Build history of the part. All positions in model axes, mm. A direction names the side the tool comes from. Give positions to 0.01 mm unless a question says otherwise; leave off trailing zeros. Loops run counter-clockwise (first coordinate to the right, second up) from the corner with the lowest first, then second, coordinate; pieces in that order, holes last.
1) Wall check: line 1 (Z direction, x = -69.85, y = -1.05); line 2 (Z direction, x = -69, y = -2); line 3 (Z direction, x = 20, y = -34.5). Give the ranges that are in metal, low to high.
2) Band-saw the part on A-A on x = -7. List the corners of the cut face in (y, z) (3 decimals).
3) Flat gauge pins, fed straight in: P1, Ø8, axis at x = -47, z = 7, coming from the -Y side (3 decimals); P2, Ø10, axis at x = 16, y = -18, coming from the -Z side; P3, Ø1, axis at x = 0.5, y = -1, coming from the +Z side. Where does each tip first touch, or does it go through?
4) Band-saw the part on B-B on y = -7. List the corners of the cut face in (x, z).
5) Two-plate mould, pull along X, no slides. Class faces 3 (the flat face through (1, -38, 95.109)), 4 (the flat face through (-77.712, -1, 43)), 5 (the cylindrical face through (-0.214, -9.744, 91.054)): +X half, -X half, draft (parallel to the pull), parting line (faces both ways), or undercut.
6) 3-axis set-ups, long thin cutter, end or side, ignore diameter. For faces 1 (the flat face through (1, -39, 88.736)), 2 (the flat face through (76.56, -1, 43)): which of +Z, -Z, +X, -X, +Y, -Y reach the whole face in a straight line?
7) Band-saw the part on C-C on x = 50.5. List the corners of the cut face in (y, z) (3 decimals), then the cut area to 3 significant figures.
8) Band-saw the part on D-D on z = -68. List the corners of the cut face in (x, y) (3 decimals), then the cut area to 3 significant figures.
```python
from build123d import *

# Parameters (mm, degrees)
F1_DEPTH = 3.175
F2_W     = 154.2725488544
F2_H     = 6.3731148839
F3_DEPTH = 76.2
F4_R     = 9.7458637612
F5_DEPTH = 25.4


with BuildPart() as f1:
    # F0 (on Front) → F1 (new body)
    with BuildSketch(Plane.XZ):
        with BuildLine():
            ThreePointArc((-69.85, 73.9775), (-72.5440768363, 80.4815768363), (-66.04, 77.7875))
            Line((-66.04, 77.7875), (0, 77.7875))
            Line((0, 77.7875), (0, 88.7359380722))
            Line((0, 88.7359380722), (-77.7124390006, 88.7359380722))
            Line((-77.7124390006, 88.7359380722), (-77.7124390006, 0))
            Line((-77.7124390006, 0), (-69.85, 0))
            Line((-69.85, 0), (-69.85, 73.9775))
        make_face()
        with BuildLine():
            Line((0, 88.7359380722), (0, 77.7875))
            Line((0, 77.7875), (66.04, 77.7875))
            ThreePointArc((66.04, 77.7875), (69.85, 81.5975), (73.66, 77.7875))
            ThreePointArc((73.66, 77.7875), (72.5440768363, 75.0934231637), (69.85, 73.9775))
            Line((69.85, 73.9775), (69.85, 0))
            Line((69.85, 0), (76.5601098537, 0))
            Line((76.5601098537, 0), (76.5601098537, 88.7359380722))
            Line((76.5601098537, 88.7359380722), (0, 88.7359380722))
        make_face()
        with BuildLine():
            Line((66.04, -77.7875), (0, -77.7875))
            Line((0, -77.7875), (0, -90.3118550777))
            Line((0, -90.3118550777), (76.5601098537, -90.3118550777))
            Line((76.5601098537, -90.3118550777), (76.5601098537, 0))
            Line((76.5601098537, 0), (69.85, 0))
            Line((69.85, 0), (69.85, -73.9775))
            ThreePointArc((69.85, -73.9775), (72.5440768363, -75.0934231637), (73.66, -77.7875))
            ThreePointArc((73.66, -77.7875), (69.85, -81.5975), (66.04, -77.7875))
        make_face()
        with BuildLine():
            Line((-69.85, -73.9775), (-69.85, 0))
            Line((-69.85, 0), (-77.7124390006, 0))
            Line((-77.7124390006, 0), (-77.7124390006, -90.3118550777))
            Line((-77.7124390006, -90.3118550777), (0, -90.3118550777))
            Line((0, -90.3118550777), (0, -77.7875))
            Line((0, -77.7875), (-66.04, -77.7875))
            ThreePointArc((-66.04, -77.7875), (-72.5440768363, -80.4815768363), (-69.85, -73.9775))
        make_face()
        with BuildLine():
            Line((0, 0), (-69.85, 0))
            Line((-69.85, 0), (-69.85, -73.9775))
            ThreePointArc((-69.85, -73.9775), (-67.1559231637, -75.0934231637), (-66.04, -77.7875))
            Line((-66.04, -77.7875), (0, -77.7875))
            Line((0, -77.7875), (0, 0))
        make_face()
        with BuildLine():
            Line((0, 77.7875), (-66.04, 77.7875))
            ThreePointArc((-66.04, 77.7875), (-67.1559231637, 75.0934231637), (-69.85, 73.9775))
            Line((-69.85, 73.9775), (-69.85, 0))
            Line((-69.85, 0), (0, 0))
            Line((0, 0), (0, 77.7875))
        make_face()
        with BuildLine():
            Line((66.04, 77.7875), (0, 77.7875))
            Line((0, 77.7875), (0, 0))
            Line((0, 0), (69.85, 0))
            Line((69.85, 0), (69.85, 73.9775))
            ThreePointArc((69.85, 73.9775), (67.1559231637, 75.0934231637), (66.04, 77.7875))
        make_face()
        with BuildLine():
            Line((69.85, 0), (0, 0))
            Line((0, 0), (0, -77.7875))
            Line((0, -77.7875), (66.04, -77.7875))
            ThreePointArc((66.04, -77.7875), (67.1559231637, -75.0934231637), (69.85, -73.9775))
            Line((69.85, -73.9775), (69.85, 0))
        make_face()
    extrude(amount=F1_DEPTH)

    # F2 (on face) → F3 (join)
    with BuildSketch(Plane(origin=(0, 0, 0), x_dir=(-1, 0, 0), z_dir=(0, 1, 0))):
        with Locations((0.5761645734, 91.9224955142)):
            Rectangle(F2_W, F2_H)
    extrude(amount=-F3_DEPTH)

    # F4 (on face) → F5 (cut)
    with BuildSketch(Plane.XY.offset(95.1090529561)):
        Circle(F4_R)
    extrude(amount=-F5_DEPTH, mode=Mode.SUBTRACT)


solid = f1.part
```
Findings below:
1. line 1: z = -90.31 to -81.6, -73.98 to 73.98, 81.6 to 95.11
1. line 2: z = -90.31 to -81.5, -74.07 to 74.07, 81.5 to 95.11
1. line 3: z = 88.74 to 95.11
2. outline: (-76.2, 88.736) - (-6.781, 88.736) - (-6.781, 95.109) - (-76.2, 95.109) - close; (-3.175, -90.312) - (0, -90.312) - (0, 69.709) - (-3.175, 69.709) - close
3. P1: stops at y = -3.175
3. P2: stops at z = 88.74
3. P3: stops at z = 69.71
4. outline: (-77.71, 88.74) - (-6.78, 88.74) - (-6.78, 95.11) - (-77.71, 95.11) - close; (6.78, 88.74) - (76.56, 88.74) - (76.56, 95.11) - (6.78, 95.11) - close
5. face 3: draft
5. face 4: -X half
5. face 5: undercut
6. face 1: -Z, +X, -X, -Y
6. face 2: +Z, -Z, +X, +Y, -Y
7. outline: (-76.2, 88.736) - (-3.175, 88.736) - (-3.175, -90.312) - (0, -90.312) - (0, 95.109) - (-76.2, 95.109) - close
7. area: 1,050 mm2
8. outline: (-77.712, -3.175) - (76.56, -3.175) - (76.56, 0) - (-77.712, 0) - close
8. area: 490 mm2
